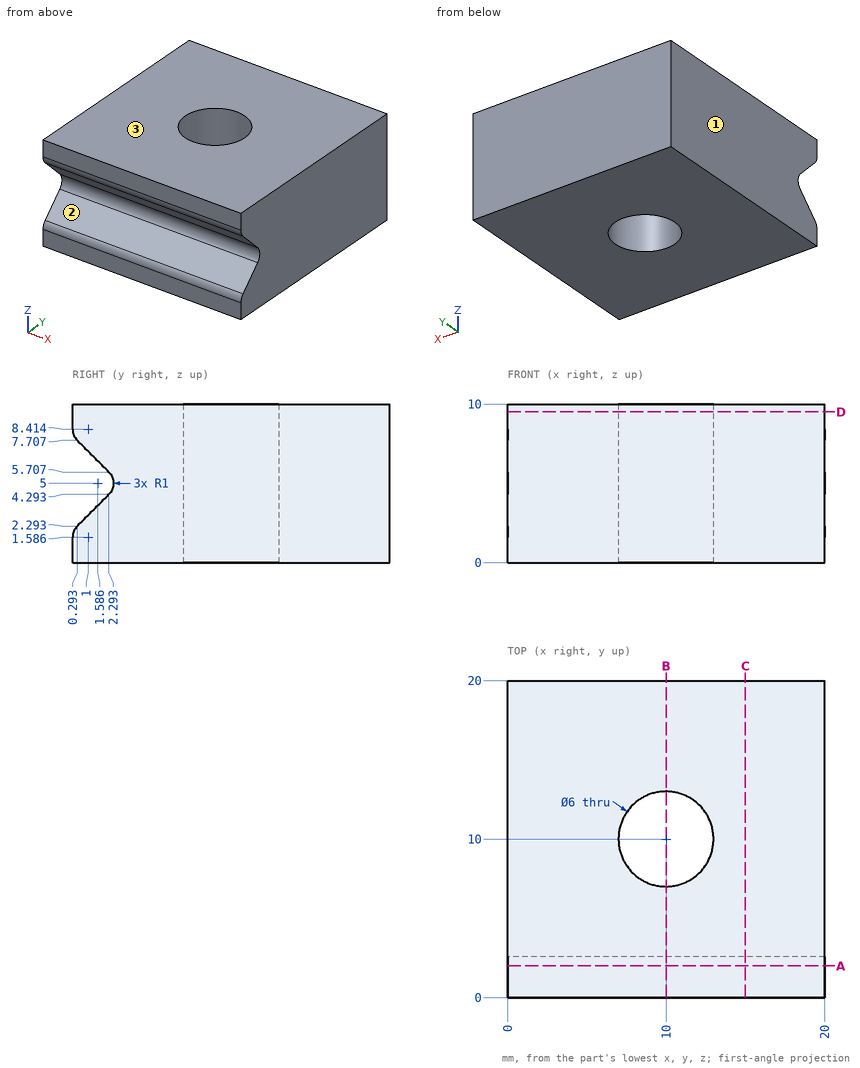
Drawing for the job (mm, zero at the part's lowest x, y, z). Coordinates: 2 decimals unless noted, no trailing zeros. Write each loop counter-clockwise with the first axis right and the second up, starting at its lowest first coordinate (ties: lowest second). Pieces come first, ordered by that corner, then holes. Notation, with made-up numbers: (43, 8) - (62, 8) arc R20 ccw to (62, 23) - close; hole circle Ø4 at (-16, -22). An arc over 180 degrees is marked (long way). Write each question's results on one line, items separated by ' | '. Start each with the question number.
1) Cut at D-D (z = 9.5). Write the cut outline in (x, y), then the cut area to 3 significant figures.
2) Mould opens along Z. For the marked faces 1, 2 and 3 say: pulls with the +Z half, pulls with the -Z half, needs draft (parallel to the pull), parting line crosses it, or undercut.
3) Cut at A-A (y = 2). Write the cut outline in (x, z).
4) Cut at B-B (x = 10). Write the cut outline in (y, z), then the cut area to 3 significant figures.
5) Probe line 1 along X through (y, z) = (12.25, 2.5) (1 decimal); line 2 along Y through (x, z) = (10, 6.75); line 3 along Y through (x, z) = (16.5, 5). List the from-to ranges inside material, lowest first. Write a range as from..to.
6) Cut at C-C (x = 15). Write the cut outline in (y, z).
Returned:
1) outline: (0, 0) - (20, 0) - (20, 20) - (0, 20) - close; hole circle Ø6 at (10, 10) | area: 372 mm^2
2) face 1: needs draft | face 2: undercut | face 3: pulls with the +Z half
3) outline: (0, 0) - (20, 0) - (20, 4) - (0, 4) - close; (0, 6) - (20, 6) - (20, 10) - (0, 10) - close
4) outline: (0, 0) - (7, 0) - (7, 10) - (0, 10) - (0, 8.41) arc R1 ccw to (0.29, 7.71) - (2.29, 5.71) arc R1 cw to (2.29, 4.29) - (0.29, 2.29) arc R1 ccw to (0, 1.59) - close; (13, 0) - (20, 0) - (20, 10) - (13, 10) - close | area: 131 mm^2
5) line 1: 0..8, 12..20 | line 2: 1.25..7, 13..20 | line 3: 2.59..20
6) outline: (0, 0) - (20, 0) - (20, 10) - (0, 10) - (0, 8.41) arc R1 ccw to (0.29, 7.71) - (2.29, 5.71) arc R1 cw to (2.29, 4.29) - (0.29, 2.29) arc R1 ccw to (0, 1.59) - close
